```python
from build123d import *

# Parameters (mm, degrees)
SKETCH1_R           = 31.75
BOSS_EXTRUDE1_DEPTH = 2
SKETCH3_R           = 12.35
BOSS_EXTRUDE3_DEPTH = 4.25
CUT_EXTRUDE1_DEPTH  = 47.608743815


with BuildPart() as part:
    # Sketch1 → Boss-Extrude1 (new body)
    with BuildSketch(Plane.XY):
        Circle(SKETCH1_R)
        with BuildLine():
            Line((1.5, 12.258568432), (1.5, 21.297241605))
            ThreePointArc((1.5, 21.297241605), (0, 21.35), (-1.5, 21.297241605))
            Line((-1.5, 21.297241605), (-1.5, 12.258568432))
            ThreePointArc((-1.5, 12.258568432), (0, 12.35), (1.5, 12.258568432))
        make_face(mode=Mode.SUBTRACT)
        with BuildLine():
            Line((-12.258568432, 1.5), (-21.297241605, 1.5))
            ThreePointArc((-21.297241605, 1.5), (-21.35, 0), (-21.297241605, -1.5))
            Line((-21.297241605, -1.5), (-12.258568432, -1.5))
            ThreePointArc((-12.258568432, -1.5), (-12.35, 0), (-12.258568432, 1.5))
        make_face(mode=Mode.SUBTRACT)
        with BuildLine():
            Line((-1.5, -12.258568432), (-1.5, -21.297241605))
            ThreePointArc((-1.5, -21.297241605), (0, -21.35), (1.5, -21.297241605))
            Line((1.5, -21.297241605), (1.5, -12.258568432))
            ThreePointArc((1.5, -12.258568432), (0, -12.35), (-1.5, -12.258568432))
        make_face(mode=Mode.SUBTRACT)
        with BuildLine():
            Line((12.258568432, -1.5), (21.297241605, -1.5))
            ThreePointArc((21.297241605, -1.5), (21.35, 0), (21.297241605, 1.5))
            Line((21.297241605, 1.5), (12.258568432, 1.5))
            ThreePointArc((12.258568432, 1.5), (12.35, 0), (12.258568432, -1.5))
        make_face(mode=Mode.SUBTRACT)
    extrude(amount=BOSS_EXTRUDE1_DEPTH)

    # Sketch3 → Boss-Extrude3 (add)
    with BuildSketch(Plane.XY.offset(2)):
        with Locations(Location((0, 0, 0), (0, 0, 173.023774077))):
            Circle(SKETCH3_R)
    extrude(amount=BOSS_EXTRUDE3_DEPTH)

    # Mirror1: part across plane


with BuildPart() as part_1:
    add(part.part)
    add(part.part.mirror(Plane.XY.offset(6.25)))

    # Sketch4 → Cut-Extrude1 (cut, through all)
    with BuildSketch(Plane(origin=(0, 0, 0), x_dir=(-1, 0, 0), z_dir=(0, 0, -1))):
        with BuildLine():
            Line((1, 6.683748948), (1, 9.296370259))
            ThreePointArc((1, 9.296370259), (0, 9.35), (-1, 9.296370259))
            Line((-1, 9.296370259), (-1, 6.683748948))
            ThreePointArc((-1, 6.683748948), (-1.109651101, 6.371294572), (-1.390510949, 6.195884061))
            ThreePointArc((-1.390510949, 6.195884061), (-5.499261314, 3.175), (-6.06104847, -1.893724225))
            ThreePointArc((-6.06104847, -1.893724225), (-6.072528505, -2.224661243), (-6.288296381, -2.47584907))
            Line((-6.288296381, -2.47584907), (-8.550892808, -3.782159726))
            ThreePointArc((-8.550892808, -3.782159726), (-8.097337525, -4.675), (-7.550892808, -5.514210533))
            Line((-7.550892808, -5.514210533), (-5.288296381, -4.207899878))
            ThreePointArc((-5.288296381, -4.207899878), (-4.962877404, -4.146633329), (-4.670537522, -4.302159837))
            ThreePointArc((-4.670537522, -4.302159837), (0, -6.35), (4.670537522, -4.302159837))
            ThreePointArc((4.670537522, -4.302159837), (4.962877404, -4.146633329), (5.288296381, -4.207899878))
            Line((5.288296381, -4.207899878), (7.550892808, -5.514210533))
            ThreePointArc((7.550892808, -5.514210533), (8.097337525, -4.675), (8.550892808, -3.782159726))
            Line((8.550892808, -3.782159726), (6.288296381, -2.47584907))
            ThreePointArc((6.288296381, -2.47584907), (6.072528505, -2.224661243), (6.06104847, -1.893724225))
            ThreePointArc((6.06104847, -1.893724225), (5.499261314, 3.175), (1.390510949, 6.195884061))
            ThreePointArc((1.390510949, 6.195884061), (1.109651101, 6.371294572), (1, 6.683748948))
        make_face()
    extrude(amount=-CUT_EXTRUDE1_DEPTH, mode=Mode.SUBTRACT)


solid = part_1.part
```
Work out the finished part from the listing and answer in its coordinate system (mm). A direction names the side the tool comes from. Round coordinates to 2 decimals unless told otherwise and drop trailing zeros. Loops run counter-clockwise (first coordinate to the right, second up) from the corner with the lowest first, then second, coordinate; pieces in that order, holes last. Notation, with made-up numbers: M 85,61 L 140,61 A26 ccw 140,96 Z; hole C 85,50.5 d6. An arc over 180 degrees is marked long. Use CSV: the item, a comma, the result in double quotes.
Q1. Consider L1, parallel to Z at x = -21, y = 4.5; L2, parallel to Y at x = 17, z = 1.5. Determine where each line is inside the solid, lowest interval first.
Determined:
L1,"0 to 2, 10.5 to 12.5"
L2,"-26.82 to -1.5, 1.5 to 26.82"
Q2. The mould has two halves that part along Y. Classify faces 4 (the flat face through (14, -7, 10.5)), 5 (the cylindrical face through (-6.883, -30.995, 0.986)), 6 (the cylindrical face through (-21.35, 0.02, 11.51)): pulls with the +Y half, pulls with the -Y half, needs draft (parallel to the pull), parting line crosses it, or undercut.
Determined:
face 4,"needs draft"
face 5,"parting line crosses it"
face 6,"undercut"
Q3. Section A-A, the plane y = 0 is taken. Determine the outline of the cut face in (x, z).
Determined:
outline,"M -31.75,0 L -21.35,0 L -21.35,2 L -31.75,2 Z; M -31.75,10.5 L -21.35,10.5 L -21.35,12.5 L -31.75,12.5 Z; M -12.35,0 L -6.35,0 L -6.35,12.5 L -12.35,12.5 Z; M 6.35,0 L 12.35,0 L 12.35,12.5 L 6.35,12.5 Z; M 21.35,0 L 31.75,0 L 31.75,2 L 21.35,2 Z; M 21.35,10.5 L 31.75,10.5 L 31.75,12.5 L 21.35,12.5 Z"
Q4. Section D-D, the plane y = -23 is taken. Determine the outline of the cut face in (x, z), then the cut area to 3 significant figures.
Determined:
outline,"M -21.89,0 L 21.89,0 L 21.89,2 L -21.89,2 Z; M -21.89,10.5 L 21.89,10.5 L 21.89,12.5 L -21.89,12.5 Z"
area,"175 mm2"
Q5. Each of these flat-tipped pins is pushed along its axis until it touches: pin 1 (0.8 mm diameter, centred on y = 8, z = 5, fed in from -X); pin 2 (0.6 mm diameter, centred on y = -17.5, z = 1, fed in from +X); pin 3 (1.6 mm diameter, centred on x = -18, z = 12, fed in from -Y). Where does it stop, or does it pass through?
Determined:
pin 1,"x = -9.73"
pin 2,"x = 26.69"
pin 3,"y = -26.69"
Q6. Section B-B, the plane x = 0 is taken. Determine the outline of the cut face in (y, z), then the cut area to 3 significant figures.
Determined:
outline,"M -31.75,0 L -21.35,0 L -21.35,2 L -31.75,2 Z; M -31.75,10.5 L -21.35,10.5 L -21.35,12.5 L -31.75,12.5 Z; M -12.35,0 L -6.35,0 L -6.35,12.5 L -12.35,12.5 Z; M 9.35,0 L 12.35,0 L 12.35,12.5 L 9.35,12.5 Z; M 21.35,0 L 31.75,0 L 31.75,2 L 21.35,2 Z; M 21.35,10.5 L 31.75,10.5 L 31.75,12.5 L 21.35,12.5 Z"
area,"196 mm2"
Q7. Section C-C, the plane x = -19 is taken. Determine the outline of the cut face in (y, z).
Determined:
outline,"M -25.44,0 L -1.5,0 L -1.5,2 L -25.44,2 Z; M -25.44,10.5 L -1.5,10.5 L -1.5,12.5 L -25.44,12.5 Z; M 1.5,0 L 25.44,0 L 25.44,2 L 1.5,2 Z; M 1.5,10.5 L 25.44,10.5 L 25.44,12.5 L 1.5,12.5 Z"
Q8. A tool of negligible diameter and unlimited length cuts with its end or side. For faces 1 (the cylindrical face through (21.35, -0.02, 11.51)), 2 (the flat face through (0, -7, 0)), 3 (the flat face through (14, -7, 2)), from which of +Z, -Z, +X, -X, +Y, -Y can it reach the whole face along a straight path? Write none if from no direction.
Determined:
face 1,"+Z, -Z"
face 2,"-Z, +X, -X, +Y, -Y"
face 3,"none"
